from build123d import *

# Parameters (mm, degrees)
SKETCH2_W                = 5
SKETCH2_H                = 5
BOSS_EXTRUDE1_DEPTH      = 2
BOSS_EXTRUDE3_DEPTH      = 5
BOSS_EXTRUDE4_DEPTH      = 5
SKETCH12_W               = 5
SKETCH12_H               = 0.5
BOSS_EXTRUDE5_DEPTH      = 1
SKETCH13_W               = 0.5
SKETCH13_H               = 5
BOSS_EXTRUDE6_DEPTH      = 1
MIRROR8_COPY_1_SKETCH_W  = 5
MIRROR8_COPY_1_SKETCH_H  = 0.5
MIRROR8_COPY_1_DEPTH     = 1
MIRROR9_COPY_1_DEPTH     = 5
MIRROR14_COPY_1_SKETCH_W = 0.5
MIRROR14_COPY_1_SKETCH_H = 5
MIRROR14_COPY_1_DEPTH    = 1
BOSS_EXTRUDE7_DEPTH      = 5


with BuildPart() as part:
    # Sketch2 → Boss-Extrude1 (new body)
    with BuildSketch(Plane.XY):
        Rectangle(SKETCH2_W, SKETCH2_H)
    boss_extrude1 = extrude(amount=BOSS_EXTRUDE1_DEPTH)

    # Sketch4 → Boss-Extrude3 (add)
    with BuildSketch(Plane(origin=(2.5, 0, 0), x_dir=(0, 0, -1), z_dir=(1, 0, 0))):
        Polygon((-1.25, -2.5), (-2.741508092, -3.991508092), (-2.741508092, -4.491508092), (-0.75, -2.5), align=None)
    boss_extrude3 = extrude(amount=-BOSS_EXTRUDE3_DEPTH)

    # Sketch9 → Boss-Extrude4 (add)
    with BuildSketch(Plane(origin=(0, 2.5, 0), x_dir=(1, 0, 0), z_dir=(0, 1, 0))):
        Polygon((2.5, -0.754950985), (4.519335319, -2.734295506), (4.019335319, -2.734295506), (2.5, -1.245049015), align=None)
    boss_extrude4 = extrude(amount=-BOSS_EXTRUDE4_DEPTH)

    # Mirror2: Boss-Extrude3 across plane
    add(boss_extrude3.mirror(Plane.ZX))

    # Mirror3: Boss-Extrude4 across plane
    add(boss_extrude4.mirror(Plane(origin=(0, 0, 0), x_dir=(0, 0, 1), z_dir=(1, 0, 0))))

    # Sketch12 → Boss-Extrude5 (add)
    with BuildSketch(Plane.XY.offset(2.741508092)):
        with Locations((0, -4.241508092)):
            Rectangle(SKETCH12_W, SKETCH12_H)
    boss_extrude5 = extrude(amount=BOSS_EXTRUDE5_DEPTH)

    # Sketch13 → Boss-Extrude6 (add)
    with BuildSketch(Plane.XY.offset(2.734295506)):
        with Locations((4.269335319, 0)):
            Rectangle(SKETCH13_W, SKETCH13_H)
    boss_extrude6 = extrude(amount=BOSS_EXTRUDE6_DEPTH)

    # Mirror4: Boss-Extrude5 across plane
    add(boss_extrude5.mirror(Plane.ZX))

    # Mirror5: Boss-Extrude6 across plane
    add(boss_extrude6.mirror(Plane(origin=(0, 0, 0), x_dir=(0, 0, 1), z_dir=(1, 0, 0))))

    # Mirror8: Boss-Extrude5 across plane
    add(boss_extrude5.mirror(Plane.XY.offset(3.741508092)))

    # Mirror8 copy 1 sketch → Mirror8 copy 1 (add)
    with BuildSketch(Plane(origin=(0, 0, 4.741508092), x_dir=(1, 0, 0), z_dir=(0, 0, -1))):
        with Locations((0, -4.241508092)):
            Rectangle(MIRROR8_COPY_1_SKETCH_W, MIRROR8_COPY_1_SKETCH_H)
    extrude(amount=MIRROR8_COPY_1_DEPTH)

    # Mirror9: Boss-Extrude3 across plane
    add(boss_extrude3.mirror(Plane.XY.offset(3.741508092)))

    # Mirror9 copy 1 sketch → Mirror9 copy 1 (add)
    with BuildSketch(Plane(origin=(2.5, 0, 7.483016184), x_dir=(0, 0, 1), z_dir=(1, 0, 0))):
        Polygon((-1.25, -2.5), (-2.741508092, -3.991508092), (-2.741508092, -4.491508092), (-0.75, -2.5), align=None)
    extrude(amount=-MIRROR9_COPY_1_DEPTH)

    # Mirror14: Boss-Extrude6 across plane
    add(boss_extrude6.mirror(Plane.XY.offset(3.734295506)))

    # Mirror14 copy 1 sketch → Mirror14 copy 1 (add)
    with BuildSketch(Plane(origin=(0, 0, 4.734295506), x_dir=(-1, 0, 0), z_dir=(0, 0, -1))):
        with Locations((4.269335319, 0)):
            Rectangle(MIRROR14_COPY_1_SKETCH_W, MIRROR14_COPY_1_SKETCH_H)
    extrude(amount=MIRROR14_COPY_1_DEPTH)

    # Sketch14 → Boss-Extrude7 (add)
    with BuildSketch(Plane.XZ.offset(2.5)):
        Polygon((4.519335319, 4.734295506), (4.019335319, 4.734295506), (2.508072629, 6.215629239), (2.508072629, 6.705727268), align=None)
    boss_extrude7 = extrude(amount=-BOSS_EXTRUDE7_DEPTH)

    # Mirror15: Boss-Extrude7 across plane
    add(boss_extrude7.mirror(Plane(origin=(0, 0, 0), x_dir=(0, 0, 1), z_dir=(1, 0, 0))))

    # Mirror16: Boss-Extrude1 across plane
    add(boss_extrude1.mirror(Plane.XY.offset(3.741508092)))


solid = part.part
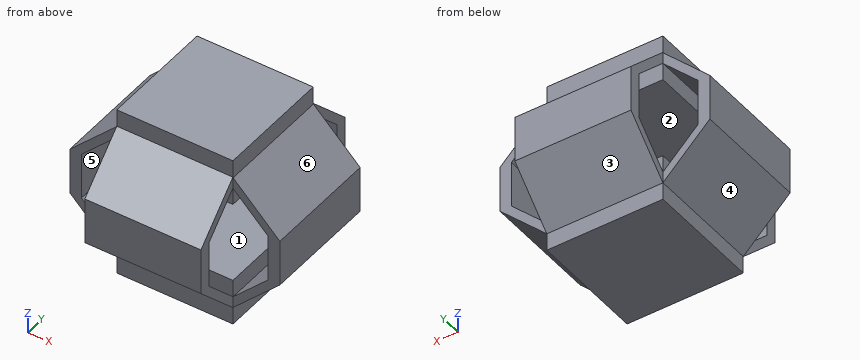
Verification items for the finished model (mm, model axes). Face numbers are marked on the shaded views. A direction names the side the tool comes from. Coordinates: 2 decimals unless noted, no trailing zeros. Loops run counter-clockwise (first coordinate to the right, second up) from the corner with the lowest first, then second, coordinate; pieces in that order, holes last. Notation, with made-up numbers: (-10.75, 13) -> (18.25, 13) arc R31 cw to (18.25, 37) -> close; hole circle Ø7 at (32.25, 11.25). An arc over 180 degrees is marked (long way). Answer as a JSON object with one key per item and string values. Group by question number.
Item 1: Mould release check, pull along Y, two halves, no side actions. Record for the marked faces 1, 2, 3 and 4: +Y half, -Y half, draft (parallel to the pull), parting line (faces both ways), or undercut.
Item 2: Sectioned sample at A-A on y = -1.5. Record the boundary of the cut face in (x, z), plus the area to 3 significant figures.
Item 3: Tool access check on the marked faces 5 and 6. Record the directions out of +Z, -Z, +X, -X, +Y, -Y that give a thin tool (end or side, any length) a straight path to the whole face; none if there is none.
Item 4: Sectioned sample at C-C on x = 2.25. Record the boundary of the cut face in (y, z).
Item 5: Sectioned sample at D-D on z = 6. Record the boundary of the cut face in (x, y), plus the area to 3 significant figures.
Item 6: Sectioned sample at B-B on z = 4.25. Record the boundary of the cut face in (x, y).
Item 7: Scan lines: probe 1 along Y at (x, z) = (-0.5, 4.25); probe 2 along Z at (x, y) = (1.5, 0); probe 3 along Y at (x, z) = (-0.5, 1.75). Record each from-to range of solid material in increasing order.
Item 8: Depth check by flat-ended pin: pin 1 (2 mm diameter, centred on x = -3, z = 3, fed in from +Y); pin 2 (0.8 mm diameter, centred on x = -1, z = 0.5, fed in from +Y); pin 3 (1 mm diameter, centred on x = -2, z = 1, fed in from -Y); pin 4 (0.6 mm diameter, centred on x = 0, z = 6, fed in from +Y). Enter the tip coordinate at first touch or a pass-through.
Evaluation:
{
 "1": {"face 1": "undercut", "face 2": "undercut", "face 3": "+Y half", "face 4": "draft"},
 "2": {"outline": "(-4.52, 2.73) -> (-2.5, 0.75) -> (-2.5, 0) -> (2.5, 0) -> (2.5, 0.75) -> (4.52, 2.73) -> (4.52, 4.73) -> (2.51, 6.71) -> (2.51, 6.22) -> (4.02, 4.73) -> (4.02, 2.73) -> (2.5, 1.25) -> (2.5, 2) -> (-2.5, 2) -> (-2.5, 1.25) -> (-4.02, 2.73) -> (-4.02, 4.73) -> (-2.51, 6.22) -> (-2.51, 6.71) -> (-4.52, 4.73) -> close; (-2.5, 5.48) -> (2.5, 5.48) -> (2.5, 7.48) -> (-2.5, 7.48) -> close", "area": "25.5 mm²"},
 "3": {"face 5": "+Y, -Y", "face 6": "+Z, +X, +Y, -Y"},
 "4": {"outline": "(-4.49, 2.74) -> (-2.5, 0.75) -> (-2.5, 0) -> (2.5, 0) -> (2.5, 0.75) -> (4.49, 2.74) -> (4.49, 4.74) -> (2.5, 6.73) -> (2.5, 7.48) -> (-2.5, 7.48) -> (-2.5, 6.73) -> (-4.49, 4.74) -> close; hole (-3.99, 2.74) -> (-2.5, 1.25) -> (-2.5, 2) -> (2.5, 2) -> (2.5, 1.25) -> (3.99, 2.74) -> (3.99, 4.74) -> (2.5, 6.23) -> (2.5, 5.48) -> (-2.5, 5.48) -> (-2.5, 6.23) -> (-3.99, 4.74) -> close"},
 "5": {"outline": "(-3.23, -2.5) -> (-2.73, -2.5) -> (-2.73, 2.5) -> (-3.23, 2.5) -> close; (-2.5, -3.23) -> (2.5, -3.23) -> (2.5, -2.73) -> (-2.5, -2.73) -> close; (-2.5, -2.5) -> (2.5, -2.5) -> (2.5, 2.5) -> (-2.5, 2.5) -> close; (-2.5, 2.73) -> (2.5, 2.73) -> (2.5, 3.23) -> (-2.5, 3.23) -> close; (2.73, -2.5) -> (3.23, -2.5) -> (3.23, 2.5) -> (2.73, 2.5) -> close", "area": "35.0 mm²"},
 "6": {"outline": "(-4.52, -2.5) -> (-4.02, -2.5) -> (-4.02, 2.5) -> (-4.52, 2.5) -> close; (-2.5, -4.49) -> (2.5, -4.49) -> (2.5, -3.99) -> (-2.5, -3.99) -> close; (-2.5, 3.99) -> (2.5, 3.99) -> (2.5, 4.49) -> (-2.5, 4.49) -> close; (4.02, -2.5) -> (4.52, -2.5) -> (4.52, 2.5) -> (4.02, 2.5) -> close"},
 "7": {"probe 1": "y = -4.49 to -3.99, 3.99 to 4.49", "probe 2": "z = 0 to 2, 5.48 to 7.48", "probe 3": "y = -3.5 to -3, -2.5 to 2.5, 3 to 3.5"},
 "8": {"pin 1": "stops at y = 4.49", "pin 2": "stops at y = 2.65", "pin 3": "stops at y = -3.25", "pin 4": "stops at y = 3.53"}
}
